Autodesk Inventor part; units mm, degrees
ref_plane "YZ Plane" through (0, 0, 0) normal (1, 0, 0) x (0, 1, 0)
ref_plane "XZ Plane" through (0, 0, 0) normal (0, 1, 0) x (-1, 0, 0)
ref_plane "XY Plane" through (0, 0, 0) normal (0, 0, 1) x (1, 0, 0)
sketch "Sketch1" plane through (0, 0, 0) normal (0, 0, 1) x (1, 0, 0)
  circle A0 centre (30.5438, 1.69) radius 1.7
  circle A1 centre (48.2215, -15.9877) radius 1.7
  line L0 (20.3327, -25.9449) -> (20.3327, 11.6471)
  circle A2 centre (39.3827, -7.1489) radius 7.62
  line L1 (39.3827, -7.1489) -> (121.2052, -7.1489) construction
  line L2 (20.3327, 11.9011) -> (58.4327, 11.9011)
  line L3 (39.3827, -7.1489) -> (118.6167, -7.1489) construction
  circle A3 centre (65.1936, -44.0106) radius 7.62
  line L4 (20.3327, 11.9011) -> (90.1827, 11.9011)
  line L5 (90.1827, 11.9011) -> (90.1827, -64.2989)
  line L6 (90.1827, -64.2989) -> (20.3327, -64.2989)
  line L7 (20.3327, -64.2989) -> (20.3327, 11.9011)
  circle A4 centre (65.1936, -44.0106) radius 18.9992
  line L8 (39.3827, -7.1489) -> (98.3795, -91.4051)
  line L9 (39.3827, -7.1489) -> (142.2405, -7.1489) construction
  line L10 (77.3997, -64.2989) -> (39.3827, -64.2989)
  line L11 (20.5867, 11.9011) -> (58.1787, 11.9011)
  line L12 (84.3087, -63.0098) -> (46.1944, -63.0098)
  line L13 (84.3087, -24.9302) -> (84.3087, -63.0098)
  line L14 (20.3327, -26.1989) -> (46.1944, -63.0098)
  line L15 (58.4327, 11.9011) -> (84.3087, -24.9302)
  point P0 (0, 0)
  dimension "d3" = 15.24
  dimension "d14" = 10.2112
  dimension "d17" = 27.8888
  dimension "d36" = 38.1
  dimension "d42" = 15.24
  dimension "d43" = 44.9999
  dimension "d51" = 69.85
  dimension "d52" = 76.2
  dimension "d53" = 37.9984
  dimension "d54" = 55
  dimension "d55" = 0
  dimension "d56" = 19.05
  dimension "d57" = 19.05
  dimension "d58" = 0
extrude "Extrusion6" add sketch "Sketch1" along normal blind 3.175 contours L0 L7 L2 L15 L13 L12 L8 A4 L14 | A4 L8 A3 | A4 L8 L12 | A4 L8 A3
equation "\"d57\" = d56"
properties part number "Motor and gearbox panel"
The listing builds one solid part. Answer for the finished solid, in the listing's coordinates (mm). Coordinates: 2 decimals unless noted, no trailing zeros. Write each loop counter-clockwise with the first axis right and the second up, starting at its lowest first coordinate (ties: lowest second). Pieces come first, ordered by that corner, then holes. Notation, with made-up numbers: (-26.75, -35) - (3.25, -35) arc R22 ccw to (3.25, -20) - close; hole circle Ø4 at (48.5, 35.25). An arc over 180 degrees is marked (long way). Return JSON: item names as keys, results as strings.
1. For a pull along Y with two mould halves and no side action, classify faces 1 (the face through (84.309, -44, 2)), 2 (the face through (37.73, 0.29, 1.57)), 3 (the face through (66, -63.01, 2)) as +Y half, -Y half, draft (parallel to the pull), parting line (faces both ways), or undercut.
Final values:
{"face 1": "draft", "face 2": "undercut", "face 3": "-Y half"}
2. The part is cut by section B-B on y = -9.5. Determine the outline of the cut face in (x, z) (3 decimals), then the cut area to 3 significant figures.
Final values:
{"outline": "(20.333, 0) - (32.134, 0) - (32.134, 3.175) - (20.333, 3.175) - close; (46.631, 0) - (73.468, 0) - (73.468, 3.175) - (46.631, 3.175) - close", "area": "123 mm^2"}
3. The part is cut by section D-D on y = -19. Determine the outline of the cut face in (x, z) (3 decimals), then the cut area to 3 significant figures.
Final values:
{"outline": "(20.333, 0) - (80.142, 0) - (80.142, 3.175) - (20.333, 3.175) - close", "area": "190 mm^2"}
4. The part is cut by section C-C on z = 1. Determine the outline of the cut face in (x, y).
Final values:
{"outline": "(20.33, -26.2) - (46.19, -63.01) - (84.31, -63.01) - (84.31, -24.93) - (58.43, 11.9) - (20.33, 11.9) - close; hole circle Ø3.4 at (30.54, 1.69); hole circle Ø15.24 at (39.38, -7.15); hole circle Ø3.4 at (48.22, -15.99); hole circle Ø15.24 at (65.19, -44.01)"}
5. Consider line 1 along X through (y, z) = (-16.5, 1.55); line 2 along X through (y, z) = (-6.5, 2.45); line 3 along Y through (x, z) = (60, 0.4). Determine where each line is inside the solid, lowest interval first.
Final values:
{"line 1": "20.33 to 46.6, 49.84 to 78.39", "line 2": "20.33 to 31.79, 46.98 to 71.36", "line 3": "-63.01 to -49.59, -38.43 to 9.67"}
6. This flat-tipped pin is pushed along its axis until it touches: pin 1 Ø1.5 at (y, z) = (-3.5, 2) entering from +X. Where does it stop, or does it pass through?
Final values:
{"pin 1": "x = 69.78"}
7. The part is cut by section A-A on x = 42. Determine the outline of the cut face in (y, z) (1 decimal).
Final values:
{"outline": "(-57, 0) - (-14.3, 0) - (-14.3, 3.2) - (-57, 3.2) - close; (0, 0) - (11.9, 0) - (11.9, 3.2) - (0, 3.2) - close"}
